Autodesk Inventor part; units mm, degrees
ref_plane "YZ Plane" through (0, 0, 0) normal (1, 0, 0) x (0, 1, 0)
ref_plane "XZ Plane" through (0, 0, 0) normal (0, 1, 0) x (-1, 0, 0)
ref_plane "XY Plane" through (0, 0, 0) normal (0, 0, 1) x (1, 0, 0)
sketch "Sketch4" plane through (0, 0, 0) normal (0, 0, 1) x (1, 0, 0)
  line L0 (0, 0) -> (400, 0)
  line L1 (400, 0) -> (400, 300)
  line L2 (400, 300) -> (0, 300)
  line L3 (0, 300) -> (0, 0)
  dimension "d9" = 400
  dimension "d10" = 300
extrude "Plate2" add sketch "Sketch4" along normal blind 1.214
sketch "Sketch6" plane through (0, 0, 0) normal (0, 0, 1) x (1, 0, 0)
  line L0 (400, 0) -> (0, 0)
  line L1 (0, 300) -> (0, 0)
  circle A0 centre (200, 150) radius 25
  dimension "d13" = 50
extrude "Cut3" cut sketch "Sketch6" along normal blind 1.214
sketch "Sketch7" plane through (0, 0, 0) normal (0, 0, 1) x (1, 0, 0)
  line L0 (0, 0) -> (20, 0)
  line L1 (20, 0) -> (20, 20)
  line L2 (20, 20) -> (0, 20)
  line L3 (0, 20) -> (0, 0)
  dimension "d16" = 20
  dimension "d17" = 20
extrude "Cut4" cut sketch "Sketch7" along normal blind 1.214
sketch "Sketch8" plane through (0, 0, 0) normal (0, 0, 1) x (1, 0, 0)
  line L0 (400, 0) -> (400, 300)
  line L1 (400, 0) -> (380, 0)
  line L2 (380, 0) -> (380, 20)
  line L3 (380, 20) -> (400, 20)
  line L4 (400, 20) -> (400, 0)
  line L5 (400, 300) -> (380, 300)
  line L6 (380, 300) -> (380, 280)
  line L7 (380, 280) -> (400, 280)
  line L8 (400, 280) -> (400, 300)
  line L9 (400, 300) -> (0, 300)
  line L10 (0, 300) -> (20, 300)
  line L11 (20, 300) -> (20, 280)
  line L12 (20, 280) -> (0, 280)
  line L13 (0, 280) -> (0, 300)
  point P0 (0, 0)
  dimension "d20" = 20
  dimension "d21" = 20
  dimension "d22" = 20
  dimension "d23" = 20
  dimension "d24" = 20
  dimension "d25" = 20
extrude "Cut5" cut sketch "Sketch8" along normal blind 1.214
equation "\"d14\" = Thickness"
equation "\"d18\" = Thickness"
equation "\"d26\" = Thickness"
equation "\"BendRadius\" = Thickness"
equation "\"BendReliefWidth\" = Thickness"
equation "\"BendReliefDepth\" = 0.5 * Thickness"
equation "\"CornerReliefSize\" = 4 * Thickness"
equation "\"MinimumRemnant\" = 2 * Thickness"
equation "\"TransitionRadius\" = BendRadius"
equation "\"JacobiRadiusSize\" = BendRadius"
equation "\"GapSize\" = Thickness"
equation "\"d2\" = BendRadius"
equation "\"d11\" = BendRadius"
properties part number "FrameSheetLaserViewport" material "Steel, Galvanized"
The listing builds one solid part. Answer for the finished solid, in the listing's coordinates (mm). Coordinates: 2 decimals unless noted, no trailing zeros. Loops run counter-clockwise (first coordinate to the right, second up) from the corner with the lowest first, then second, coordinate; pieces in that order, holes last. Notation, with made-up numbers: (-22.5, 83) - (-10.5, 83) arc R16 ccw to (-10.5, 98) - close; hole circle Ø5 at (57.25, 66). An arc over 180 degrees is marked (long way). Use a Markdown table: item, result. Add a question column.
1) Find the intervals of material crossed by line 1 (Y direction, x = 200, z = 0.8); line 2 (X direction, y = 139.5, z = 0.45), in increasing order.
2) The mould has two halves that part along Y. Classify faces 1 (the flat face through (197, 119, 0)), 2 (the cylindrical face through (223.846, 142.491, 0.599)): released by +Y, released by -Y, zero draft, split by the parting line, or undercut.
3) The part is cut by section C-C, the plane z = 0.25. Give the vertices of the cut face in (x, y).
4) The part is cut by section B-B, the plane x = 200. Give the vertices of the cut face in (y, z).
5) Given pin 1 (0.6 mm diameter, centred on x = 388, z = 1, fed in from +Y); pin 2 (0.6 mm diameter, centred on y = 9.5, z = 0.5, fed in from -X), each flat-ended and moving along its own axis, determine where each tip first touches the part or whether it passes through.
6) The part is cut by section A-A, the plane y = 150. Give the vertices of the cut face in (x, z), and give its area (3 significant figures).
Here are the results:
| question | item | result |
|---|---|---|
| 1 | line 1 | y = 0 to 125, 175 to 300 |
| 1 | line 2 | x = 0 to 177.31, 222.69 to 400 |
| 2 | face 1 | zero draft |
| 2 | face 2 | undercut |
| 3 | outline | (0, 20) - (20, 20) - (20, 0) - (380, 0) - (380, 20) - (400, 20) - (400, 280) - (380, 280) - (380, 300) - (20, 300) - (20, 280) - (0, 280) - close; hole circle Ø50 at (200, 150) |
| 4 | outline | (0, 0) - (125, 0) - (125, 1.21) - (0, 1.21) - close; (175, 0) - (300, 0) - (300, 1.21) - (175, 1.21) - close |
| 5 | pin 1 | stops at y = 280 |
| 5 | pin 2 | stops at x = 20 |
| 6 | outline | (0, 0) - (175, 0) - (175, 1.21) - (0, 1.21) - close; (225, 0) - (400, 0) - (400, 1.21) - (225, 1.21) - close |
| 6 | area | 425 mm^2 |
